Could you check a few things on this model? Use its own coordinates, in mm. Face numbers are marked on the shaded views. Give positions to 0.01 mm unless a question says otherwise; leave off trailing zeros. Loops run counter-clockwise (first coordinate to the right, second up) from the corner with the lowest first, then second, coordinate; pieces in that order, holes last. Notation, with made-up numbers: (-30, 35.5) -> (-19, 35.5) arc R20 ccw to (-19, 57.5) -> close; hole circle Ø1 at (-20, -27.75). An arc over 180 degrees is marked (long way). Write each question's results on one line, items separated by ' | '. Start each with the question number.
Q1. If we section it at C-C, the plane x = 7: List the corners of the cut face in (y, z) for me (3 decimals).
Q2. If we section it at A-A, the plane y = 0: List the corners of the cut face in (x, z) for me (3 decimals), plus the area to 3 significant figures.
Q3. If we section it at B-B, the plane x = 0: List the corners of the cut face in (y, z) for me (3 decimals).
Q4. If we section it at D-D, the plane z = 0: List the corners of the cut face in (x, y) for me, plus the area to 3 significant figures.
Q5. We'd pull the mould along Y, two halves only. Please class the marked faces 1, 2 and 3: released by +Y, released by -Y, zero draft, split by the parting line, or undercut.
Q6. Will these pins go through, and if not, where does the flat tip stop? P1, Ø4, axis at y = 7, z = 3, coming from the +X side; P2, Ø1, axis at x = -4.5, z = 6.5, coming from the -Y side; P3, Ø3, axis at x = 9.5, z = 6.5, coming from the -Y side.
Q7. If I drill on line 1 along Y through (x, z) = (0, 7.75) (3 decimals); line 2 along Y through (x, z) = (0, 2.25); line 3 along X through (y, z) = (0, 7.5) (3 decimals), over which ranges is the centre line in solid material (lowest first)?
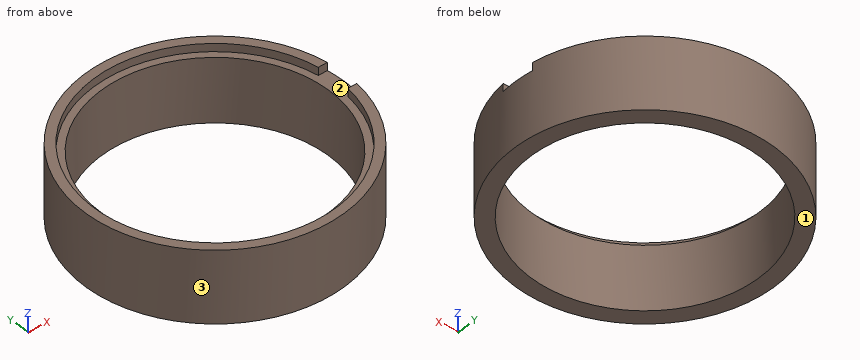
from build123d import *

# Parameters (mm, degrees)
F0_R          = 16.25
F0_R_2        = 14.25
F1_DEPTH      = 7.25
F1_DEPTH_BACK = 0.75
F2_R          = 16.25
F2_R_2        = 15.125
F3_DEPTH      = 1
F4_W          = 4
F4_H          = 4.25
F5_DEPTH      = 1


with BuildPart() as f1:
    # F0 (on Top) → F1 (new body, two sides)
    with BuildSketch(Plane.XY) as f1_sk:
        Circle(F0_R)
        Circle(F0_R_2, mode=Mode.SUBTRACT)
    extrude(amount=F1_DEPTH)
    extrude(f1_sk.sketch, amount=-F1_DEPTH_BACK)

    # F2 (on face) → F3 (join)
    with BuildSketch(Plane.XY.offset(7.25)):
        Circle(F2_R)
        Circle(F2_R_2, mode=Mode.SUBTRACT)
    extrude(amount=F3_DEPTH)

    # F4 (on face) → F5 (cut)
    with BuildSketch(Plane.XY.offset(8.25)):
        with Locations((15.125, 0)):
            Rectangle(F4_W, F4_H)
    extrude(amount=-F5_DEPTH, mode=Mode.SUBTRACT)


solid = f1.part
Final values:
1) outline: (-14.665, -0.75) -> (-12.412, -0.75) -> (-12.412, 7.25) -> (-13.408, 7.25) -> (-13.408, 8.25) -> (-14.665, 8.25) -> close; (12.412, -0.75) -> (14.665, -0.75) -> (14.665, 8.25) -> (13.408, 8.25) -> (13.408, 7.25) -> (12.412, 7.25) -> close
2) outline: (-16.25, -0.75) -> (-14.25, -0.75) -> (-14.25, 7.25) -> (-15.125, 7.25) -> (-15.125, 8.25) -> (-16.25, 8.25) -> close; (14.25, -0.75) -> (16.25, -0.75) -> (16.25, 7.25) -> (14.25, 7.25) -> close | area: 33.1 mm²
3) outline: (-16.25, -0.75) -> (-14.25, -0.75) -> (-14.25, 7.25) -> (-15.125, 7.25) -> (-15.125, 8.25) -> (-16.25, 8.25) -> close; (14.25, -0.75) -> (16.25, -0.75) -> (16.25, 8.25) -> (15.125, 8.25) -> (15.125, 7.25) -> (14.25, 7.25) -> close
4) outline: circle Ø32.5 at (0, 0); hole circle Ø28.5 at (0, 0) | area: 192 mm²
5) face 1: zero draft | face 2: undercut | face 3: split by the parting line
6) P1: stops at x = 15.46 | P2: stops at y = -15.75 | P3: stops at y = -14.14
7) line 1: y = -16.25 to -15.125, 15.125 to 16.25 | line 2: y = -16.25 to -14.25, 14.25 to 16.25 | line 3: x = -16.25 to -15.125
